Geometry check sheet. Reference: the model listing, model coordinates, mm. Give positions to 0.01 mm unless a question says otherwise; leave off trailing zeros. Loops run counter-clockwise (first coordinate to the right, second up) from the corner with the lowest first, then second, coordinate; pieces in that order, holes last. Notation, with made-up numbers: (-2, 69.25) - (6, 69.25) arc R11 ccw to (6, 84.25) - close; hole circle Ø1 at (23, -29.5). An arc over 180 degrees is marked (long way). Use a Markdown table: item, result. Add a question column.
1. Draft check along X on faces 1 (the cylindrical face through (-340.4, 171.8, 1.3)), 2 (the cylindrical face through (-365.8, 171.8, 1.3)), 3 (the flat face through (-351, 169, 2.54)), 4 (the flat face through (-334.085, 168, 1)). Enter one of: pulls with the +X half, pulls with the -X half, needs draft (parallel to the pull), parting line crosses it, or undercut.
2. Cross-section at A-A on x = -338. Enter the section's corners in (y, z).
3. Depth check by flat-ended pin: P1, Ø5.5, axis at x = -363.39, y = 171.67, coming from the +Z side; P2, Ø1, axis at x = -348, z = 1, coming from the -Y side. Enter the tip coordinate at first touch or a pass-through.
4. Cross-section at C-C on y = 172. Enter the section's corners in (x, z).
5. Cross-section at B-B on z = 2.15. Enter the section's corners in (x, y) (1 decimal), and give its area (3 significant figures).
6. Material ranges on L1, parallel to X at y = 173, z = 1.95; L2, parallel to X at y = 169.75, z = 1.7; L3, parallel to X at y = 164.5, z = 1.95, recorded low to high.
7. Cross-section at D-D on x = -353. Enter the section's corners in (y, z).
from build123d import *

# Parameters (mm, degrees)
SKETCH1_R           = 2.413
BOSS_EXTRUDE1_DEPTH = 2.54
FILLET1_R           = 2.54


with BuildPart() as part:
    # Sketch1 → Boss-Extrude1 (new body)
    # profile 1 of 2: a face of its own
    with BuildSketch(Plane.XY):
        with BuildLine():
            Line((-367.293338715, 162.140585859), (-357.133338715, 162.140585859))
            ThreePointArc((-357.133338715, 162.140585859), (-350.689077681, 168.584846892), (-344.244816647, 162.140585859))
            Line((-344.244816647, 162.140585859), (-334.084816647, 162.140585859))
            Line((-334.084816647, 162.140585859), (-334.084816647, 174.840585859))
            Line((-334.084816647, 174.840585859), (-367.293338715, 174.840585859))
            Line((-367.293338715, 174.840585859), (-367.293338715, 162.140585859))
        make_face()
        with Locations((-363.389077681, 171.665585859)):
            Circle(SKETCH1_R, mode=Mode.SUBTRACT)
        with Locations((-337.989077681, 171.665585859)):
            Circle(SKETCH1_R, mode=Mode.SUBTRACT)
    # profile 2 of 2: a face of its own
    with BuildSketch(Plane.XY):
        with BuildLine():
            ThreePointArc((-344.244816647, 162.140585859), (-350.689077681, 168.584846892), (-357.133338715, 162.140585859))
            Line((-357.133338715, 162.140585859), (-355.451577681, 162.140585859))
            ThreePointArc((-355.451577681, 162.140585859), (-350.689077681, 166.903085859), (-345.926577681, 162.140585859))
            Line((-345.926577681, 162.140585859), (-344.244816647, 162.140585859))
        make_face()
    extrude(amount=BOSS_EXTRUDE1_DEPTH)

    # Fillet1
    fillet1_edges = [part.edges().sort_by_distance(p)[0] for p in [
        (-367.293338715, 162.140585859, 1.27),
        (-367.293338715, 174.840585859, 1.27),
        (-334.084816647, 174.840585859, 1.27),
        (-334.084816647, 162.140585859, 1.27),
    ]]
    fillet(fillet1_edges, radius=FILLET1_R)


solid = part.part
Values found:
| question | item | result |
|---|---|---|
| 1 | face 1 | undercut |
| 1 | face 2 | undercut |
| 1 | face 3 | needs draft |
| 1 | face 4 | pulls with the +X half |
| 2 | outline | (162.14, 0) - (169.25, 0) - (169.25, 2.54) - (162.14, 2.54) - close; (174.08, 0) - (174.84, 0) - (174.84, 2.54) - (174.08, 2.54) - close |
| 3 | P1 | stops at z = 2.54 |
| 3 | P2 | stops at y = 165.68 |
| 4 | outline | (-367.29, 0) - (-365.78, 0) - (-365.78, 2.54) - (-367.29, 2.54) - close; (-361, 0) - (-340.38, 0) - (-340.38, 2.54) - (-361, 2.54) - close; (-335.6, 0) - (-334.08, 0) - (-334.08, 2.54) - (-335.6, 2.54) - close |
| 5 | outline | (-367.3, 164.7) arc R2.5 ccw to (-364.8, 162.1) - (-355.5, 162.1) arc R4.8 cw to (-345.9, 162.1) - (-336.6, 162.1) arc R2.5 ccw to (-334.1, 164.7) - (-334.1, 172.3) arc R2.5 ccw to (-336.6, 174.8) - (-364.8, 174.8) arc R2.5 ccw to (-367.3, 172.3) - close; hole circle Ø4.8 at (-363.4, 171.7); hole circle Ø4.8 at (-338, 171.7) |
| 5 | area | 344 mm2 |
| 6 | L1 | x = -367.2 to -365.4, -361.38 to -340, -335.98 to -334.18 |
| 6 | L2 | x = -367.29 to -364.86, -361.92 to -339.46, -336.52 to -334.08 |
| 6 | L3 | x = -367.29 to -354.83, -346.55 to -334.09 |
| 7 | outline | (166.3, 0) - (174.84, 0) - (174.84, 2.54) - (166.3, 2.54) - close |
